from build123d import *

# Parameters (mm, degrees)
F0_R     = 22.225
F0_R_2   = 17.4625
F1_DEPTH = 12.7
F2_START = 4.7625
F0_R_3   = 75.40625
F0_R_4   = 4.7625
F2_DEPTH = 4.7625
F3_R     = 3.17499


# Not quite as in the source:
# - a fillet or chamfer is up to 0.001 mm smaller than in the source, because OpenCascade refuses the exact size


with BuildPart() as f1:
    # F0 (on Front) → F1 (new body)
    with BuildSketch(Plane.XZ):
        Circle(F0_R)
        Circle(F0_R_2, mode=Mode.SUBTRACT)
    extrude(amount=F1_DEPTH)

    # F0 (on Front) → F2 (join)
    with BuildSketch(Plane.XZ.offset(F2_START)):
        Circle(F0_R_3)
        with Locations((-63.5, 0)):
            Circle(F0_R_4, mode=Mode.SUBTRACT)
        Circle(F0_R, mode=Mode.SUBTRACT)
        with Locations((63.5, 0)):
            Circle(F0_R_4, mode=Mode.SUBTRACT)
    extrude(amount=F2_DEPTH)

    # F3 (radius 3.175 in the source; OpenCascade refuses exactly that, so slightly less here)
    f3_edges = [f1.edges().sort_by_distance(p)[0] for p in [
        (-22.225, -9.525, 0),
        (-22.225, -4.7625, 0),
    ]]
    fillet(f3_edges, radius=F3_R)


solid = f1.part
Can you work these out from the model? Positions are in its coordinate system, mm. A direction names the side the tool comes from. Give positions to 0.01 mm unless a question says otherwise; leave off trailing zeros. Write each loop counter-clockwise with the first axis right and the second up, starting at its lowest first coordinate (ties: lowest second). Pieces come first, ordered by that corner, then holes. Notation, with made-up numbers: M -28.75,-19.5 L 24.25,-19.5 A9 ccw 24.25,-11.5 Z; hole C -5.5,-9.5 d3. An arc over 180 degrees is marked long. Answer in a Markdown table with one row per item. Add a question column.
Item 1: We'd pull the mould along Z, two halves only. Please class faces 1 (the cylindrical face through (-68.258, -7.11, 0.209)), 2 (the flat face through (10, -12.7, -15)), 3 (the cylindrical face through (71.924, -7.11, 22.65)): released by +Z, released by -Z, zero draft, split by the parting line, or undercut.
Item 2: Imagine slicing it at C-C, the plane y = -7.5. Write out the boundary of the cut face in (x, z) (1 decimal).
Item 3: Imagine slicing it at B-B, the plane z = 0. State how many separate pieces and enclosed holes the cut face has, plus the area to 3 significant figures.
Item 4: Imagine slicing it at D-D, the plane x = -63.5. Write out the boundary of the cut face in (y, z) (1 decimal).
Item 5: Please list where these lines run through material, in increasing order: L1, parallel to Z at x = 0, y = -9; L2, parallel to Y at x = -16, z = -61 (1 decimal); L3, parallel to Z at x = 63.5, y = -6.55.
Item 6: On a 3-axis mill with a long thin cutter (end or side, diameter ignored), from which of +Z, -Z, +X, -X, +Y, -Y can I reach the whole of each face in a straight line? I mean faces 4 (the flat face through (32, -4.762, 1)), 5 (the flat face through (32, -9.525, 1)), 6 (the flat face through (10, 0, -15)). Say none if no direction works.
Item 7: For pin 1 Ø6 at (x, y) = (-40.5, -3) entering from -Z; pin 2 Ø8 at (x, z) = (5, 52) entering from +Y; pin 3 Ø2 at (x, z) = (-0.5, -45.5) entering from -Y (3 decimals), each with a flat end and sliding along its axis, tell me the tip position at first contact or that it passes through.
Evaluation:
| question | item | result |
|---|---|---|
| 1 | face 1 | undercut |
| 1 | face 2 | zero draft |
| 1 | face 3 | split by the parting line |
| 2 | outline | C 0,0 d150.8; hole C -63.5,0 d9.5; hole C 0,0 d34.9; hole C 63.5,0 d9.5 |
| 3 | separate pieces | 4 |
| 3 | enclosed holes | 0 |
| 3 | area | 545 mm² |
| 4 | outline | M -9.5,-40.7 L -4.8,-40.7 L -4.8,-4.8 L -9.5,-4.8 Z; M -9.5,4.8 L -4.8,4.8 L -4.8,40.7 L -9.5,40.7 Z |
| 5 | L1 | z = -75.41 to -17.46, 17.46 to 75.41 |
| 5 | L2 | y = -9.5 to -4.8 |
| 5 | L3 | z = -40.67 to -4.76, 4.76 to 40.67 |
| 6 | face 4 | +Y |
| 6 | face 5 | -Y |
| 6 | face 6 | +Z, -Z, +X, -X, +Y |
| 7 | pin 1 | stops at z = -65.09 |
| 7 | pin 2 | stops at y = -4.76 |
| 7 | pin 3 | stops at y = -9.525 |
